Input: dimensioned drawing with shaded views. Units: mm. Origin: part minimum x, y, z. A direction names the side the tool comes from. Give positions to 0.01 mm unless a question says otherwise; leave off trailing zeros. Loops run counter-clockwise (first coordinate to the right, second up) from the corner with the lowest first, then second, coordinate; pieces in that order, holes last. Notation, with made-up numbers: (-18, 84) -> (0, 84) arc R27 cw to (0, 114) -> close; hole circle Ø1 at (12.5, 44). An arc over 180 degrees is marked (long way). One line per question, with ' | ' between items. Start each with the question number.
Item 1: Section A-A on z = 20. Give the number of separate pieces and of enclosed holes in the cut face.
Item 2: Section C-C on y = 22.5. Return loops of the section in (x, z).
Item 3: Pin query (flat end, axial travel): P1, Ø6.5, axis at x = 6.5, z = 20, coming from the +Y side; P2, Ø8, axis at y = 19.5, z = 10.5, coming from the +X side; P3, Ø12, axis at x = 6.5, z = 16, coming from the -Y side; P4, Ø3.5, axis at y = 6.5, z = 12, coming from the -X side (3 decimals). Return the tip coordinate at first contact, or that it passes through.
Item 4: Section D-D on y = 3. Return loops of the section in (x, z), then the cut area to 3 significant figures.
Item 5: Material intervals for line 1 along Z through (x, y) = (14.5, 1.5); line 2 along Y through (x, z) = (1.6, 12); line 3 along X through (y, z) = (1.3, 4), sorted ascending. Write a range as [from, to].
Item 6: Section B-B on x = 22.5. Return loops of the section in (y, z), then the cut area to 3 significant figures.
Item 7: Set-up query: the marked faces 1 and 2. Return all of +Z, -Z, +X, -X, +Y, -Y with unobstructed straight access to the full face (end or side cutting, diameter ignored); none if empty.
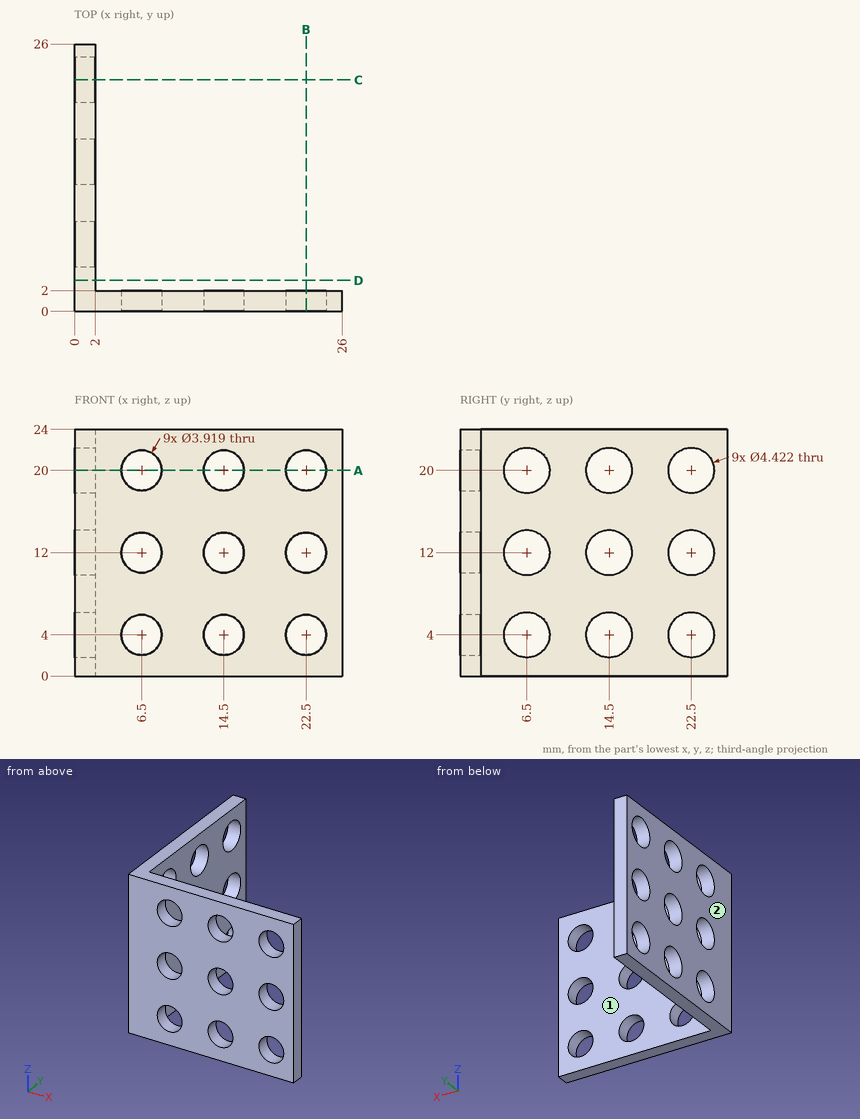
Result sheet:
1) separate pieces: 7 | enclosed holes: 0
2) outline: (0, 0) -> (2, 0) -> (2, 1.79) -> (0, 1.79) -> close; (0, 6.21) -> (2, 6.21) -> (2, 9.79) -> (0, 9.79) -> close; (0, 14.21) -> (2, 14.21) -> (2, 17.79) -> (0, 17.79) -> close; (0, 22.21) -> (2, 22.21) -> (2, 24) -> (0, 24) -> close
3) P1: stops at y = 2 | P2: stops at x = 2 | P3: stops at y = 0 | P4: passes through
4) outline: (0, 0) -> (2, 0) -> (2, 24) -> (0, 24) -> close | area: 48.0 mm²
5) line 1: z = [0, 2.04], [5.96, 10.04], [13.96, 18.04], [21.96, 24] | line 2: y = [0, 4.29], [8.71, 12.29], [16.71, 20.29], [24.71, 26] | line 3: x = [0, 4.54], [8.46, 12.54], [16.46, 20.54], [24.46, 26]
6) outline: (0, 0) -> (2, 0) -> (2, 2.04) -> (0, 2.04) -> close; (0, 5.96) -> (2, 5.96) -> (2, 10.04) -> (0, 10.04) -> close; (0, 13.96) -> (2, 13.96) -> (2, 18.04) -> (0, 18.04) -> close; (0, 21.96) -> (2, 21.96) -> (2, 24) -> (0, 24) -> close | area: 24.5 mm²
7) face 1: +Z, -Z, +X, +Y | face 2: +Z, -Z, -X, +Y, -Y
